Input: part model. Units: mm. Frame: model coordinates. Round coordinates to 2 decimals unless told otherwise and drop trailing zeros. Loops run counter-clockwise (first coordinate to the right, second up) from the corner with the lowest first, then second, coordinate; pieces in that order, holes last. Notation, with made-up numbers: M 9,69.25 L 37,69.25 A21 cw 37,77.25 Z; hole C -18.5,-35.5 d3. An arc over 180 degrees is marked long. Put each result on its own line as item: value. Start each with the question number.
1) Section B-B on x = -134.62. State how many separate pieces and enclosed holes the cut face has, plus the area to 3 significant figures.
2) Section A-A on z = -50.8. Output: boundary loops of the cut face in (x, y) (3 decimals).
3) Line query: probe 1 along Z at (x, y) = (20.32, -2.75) (3 decimals); probe 2 along X at (y, z) = (-1.25, -70); probe 3 along Z at (x, y) = (-135.5, -1.5). Output: solid intervals per line, ascending.
4) Pin query (flat end, axial travel): pin 1 (1 mm diameter, centred on y = -4, z = 78.5, fed in from +X); pin 2 (1.5 mm diameter, centred on y = -5.5, z = 68, fed in from -X). Return the tip coordinate at first contact, or that it passes through.
from build123d import *

# Parameters (mm, degrees)
F0_R     = 2.0955
F0_R_2   = 28.575
F0_R_3   = 2.1
F0_R_4   = 6.35
F0_R_5   = 3.175
F0_R_6   = 5.588
F0_R_7   = 39.6875
F0_R_8   = 1.524
F0_W     = 85
F0_H     = 55.5
F1_DEPTH = 6.35


with BuildPart() as f1:
    # F0 (on Front) → F1 (new body)
    with BuildSketch(Plane.XZ):
        with BuildLine():
            Line((-215.9, 52.07), (-215.9, -100.33))
            Line((-215.9, -100.33), (215.9, -100.33))
            Line((215.9, -100.33), (215.9, 49.53))
            add(Edge.make_bspline(
                [(85.438013, 100.33), (140.408784, 100.33), (191.265792, 74.631676), (215.9, 49.53)],
                knots=[0, 0, 0, 0, 140.003464, 140.003464, 140.003464, 140.003464], degree=3))
            Line((85.438013, 100.33), (-79.661987, 100.33))
            add(Edge.make_bspline(
                [(-79.661987, 100.33), (-174.395946, 100.33), (-194.33257, 74.093506), (-215.9, 52.07)],
                knots=[0, 0, 0, 0, 144.533124, 144.533124, 144.533124, 144.533124], degree=3))
        make_face()
        with Locations((-158.1912, -74.3712)):
            Circle(F0_R, mode=Mode.SUBTRACT)
        with Locations((-111.0488, -74.3712)):
            Circle(F0_R, mode=Mode.SUBTRACT)
        with Locations((-134.62, -50.8)):
            Circle(F0_R_2, mode=Mode.SUBTRACT)
        with Locations((-158.1912, -27.2288)):
            Circle(F0_R, mode=Mode.SUBTRACT)
        with Locations((-111.0488, -27.2288)):
            Circle(F0_R, mode=Mode.SUBTRACT)
        with Locations((-158.1912, -9.6012)):
            Circle(F0_R, mode=Mode.SUBTRACT)
        with Locations((-111.0488, -9.6012)):
            Circle(F0_R, mode=Mode.SUBTRACT)
        with Locations((-84.155, -1.2875)):
            Circle(F0_R_3, mode=Mode.SUBTRACT)
        with Locations((-21.255, -1.2875)):
            Circle(F0_R_3, mode=Mode.SUBTRACT)
        with Locations((20.32, -64.643)):
            Circle(F0_R_4, mode=Mode.SUBTRACT)
        with Locations((45.72, -64.643)):
            Circle(F0_R_4, mode=Mode.SUBTRACT)
        with Locations((71.12, -64.643)):
            Circle(F0_R_4, mode=Mode.SUBTRACT)
        with Locations((20.32, -35.18)):
            Circle(F0_R_5, mode=Mode.SUBTRACT)
        with Locations((45.72, -35.18)):
            Circle(F0_R_5, mode=Mode.SUBTRACT)
        with Locations((71.12, -35.18)):
            Circle(F0_R_5, mode=Mode.SUBTRACT)
        with Locations((20.32, -21.21)):
            Circle(F0_R_5, mode=Mode.SUBTRACT)
        with Locations((33.02, -21.21)):
            Circle(F0_R_5, mode=Mode.SUBTRACT)
        with Locations((45.72, -21.21)):
            Circle(F0_R_5, mode=Mode.SUBTRACT)
        with Locations((20.32, -7.24)):
            Circle(F0_R_5, mode=Mode.SUBTRACT)
        with Locations((58.42, -21.21)):
            Circle(F0_R_5, mode=Mode.SUBTRACT)
        with Locations((71.12, -21.21)):
            Circle(F0_R_5, mode=Mode.SUBTRACT)
        with Locations((71.12, -7.24)):
            Circle(F0_R_5, mode=Mode.SUBTRACT)
        with Locations((-176.022, 12.7)):
            Circle(F0_R_6, mode=Mode.SUBTRACT)
        with Locations((-134.62, 13.97)):
            Circle(F0_R_2, mode=Mode.SUBTRACT)
        with Locations((-176.022, 31.75)):
            Circle(F0_R_6, mode=Mode.SUBTRACT)
        with Locations((-158.1912, 37.5412)):
            Circle(F0_R, mode=Mode.SUBTRACT)
        with Locations((-111.0488, 37.5412)):
            Circle(F0_R, mode=Mode.SUBTRACT)
        with Locations((-52.705, 30.1625)):
            Circle(F0_R_7, mode=Mode.SUBTRACT)
        with Locations((-84.155, 61.6125)):
            Circle(F0_R_3, mode=Mode.SUBTRACT)
        with Locations((-21.255, 61.6125)):
            Circle(F0_R_3, mode=Mode.SUBTRACT)
        with Locations((0, 6.54)):
            Circle(F0_R_8, mode=Mode.SUBTRACT)
        with Locations((91.44, 6.54)):
            Circle(F0_R_8, mode=Mode.SUBTRACT)
        with Locations((45.72, 37.02)):
            Rectangle(F0_W, F0_H, mode=Mode.SUBTRACT)
        with Locations((0, 67.5)):
            Circle(F0_R_8, mode=Mode.SUBTRACT)
        with Locations((91.44, 67.5)):
            Circle(F0_R_8, mode=Mode.SUBTRACT)
    extrude(amount=F1_DEPTH)


solid = f1.part
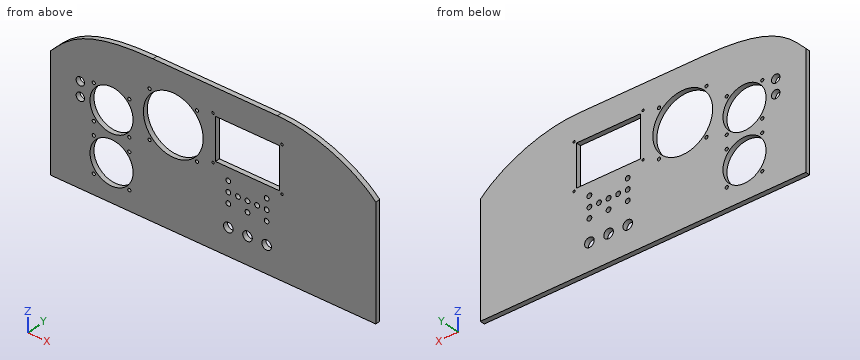
Geometry results:
1. separate pieces: 3
1. enclosed holes: 0
1. area: 524 mm²
2. outline: M -215.9,-6.35 L -163.195,-6.35 L -163.195,0 L -215.9,0 Z; M -106.045,-6.35 L 215.9,-6.35 L 215.9,0 L -106.045,0 Z
3. probe 1: z = -100.33 to -70.993, -58.293 to -38.355, -32.005 to -24.385, -18.035 to -10.415, -4.065 to 9.27, 64.77 to 100.33
3. probe 2: x = -215.9 to -155.78, -113.46 to 16.91, 23.73 to 42.31, 49.13 to 67.71, 74.53 to 215.9
3. probe 3: z = -100.33 to -79.36, -22.24 to -14.59, 42.53 to 96.3
4. pin 1: stops at x = 175.67
4. pin 2: stops at x = -200.7
